from build123d import *

# Parameters (mm, degrees)
SKETCH_1_R          = 32
EXTRUDE_1_DEPTH     = 26.5
CUT_EXTRUDE_4_DEPTH = 2
SKETCH_3_R          = 26
CUT_EXTRUDE_5_DEPTH = 1
FILLET_1_R          = 10
SKETCH_4_R          = 6.68863581
CUT_EXTRUDE_6_DEPTH = 5


with BuildPart() as part:
    # 草图1 → 凸台-拉伸1 (new body)
    with BuildSketch(Plane.XY):
        Circle(SKETCH_1_R)
    extrude(amount=EXTRUDE_1_DEPTH)

    # 草图2 → 切除-拉伸4 (cut)
    with BuildSketch(Plane.XY.offset(26.5)):
        with BuildLine():
            ThreePointArc((3.045475662, 0.479690306), (3.083022023, 0), (3.045475662, -0.479690306))
            Line((3.045475662, -0.479690306), (25.683360874, -4.045364533))
            ThreePointArc((25.683360874, -4.045364533), (26, 0), (25.683360874, 4.045364533))
            Line((25.683360874, 4.045364533), (3.045475662, 0.479690306))
        make_face()
        with BuildLine():
            Line((16.34506889, -20.219760705), (1.938161822, -2.397614137))
            ThreePointArc((1.938161822, -2.397614137), (1.541511012, -2.669975393), (1.10731384, -2.877304443))
            Line((1.10731384, -2.877304443), (9.338291984, -24.265125238))
            ThreePointArc((9.338291984, -24.265125238), (13, -22.516660498), (16.34506889, -20.219760705))
        make_face()
        with BuildLine():
            Line((-9.338291984, -24.265125238), (-1.10731384, -2.877304443))
            ThreePointArc((-1.10731384, -2.877304443), (-1.541511012, -2.669975393), (-1.938161822, -2.397614137))
            Line((-1.938161822, -2.397614137), (-16.34506889, -20.219760705))
            ThreePointArc((-16.34506889, -20.219760705), (-13, -22.516660498), (-9.338291984, -24.265125238))
        make_face()
        with BuildLine():
            Line((-25.683360874, -4.045364533), (-3.045475662, -0.479690306))
            ThreePointArc((-3.045475662, -0.479690306), (-3.083022023, 0), (-3.045475662, 0.479690306))
            Line((-3.045475662, 0.479690306), (-25.683360874, 4.045364533))
            ThreePointArc((-25.683360874, 4.045364533), (-26, 0), (-25.683360874, -4.045364533))
        make_face()
        with BuildLine():
            Line((-16.34506889, 20.219760705), (-1.938161822, 2.397614137))
            ThreePointArc((-1.938161822, 2.397614137), (-1.541511012, 2.669975393), (-1.10731384, 2.877304443))
            Line((-1.10731384, 2.877304443), (-9.338291984, 24.265125238))
            ThreePointArc((-9.338291984, 24.265125238), (-13, 22.516660498), (-16.34506889, 20.219760705))
        make_face()
        with BuildLine():
            Line((9.338291984, 24.265125238), (1.10731384, 2.877304443))
            ThreePointArc((1.10731384, 2.877304443), (1.541511012, 2.669975393), (1.938161822, 2.397614137))
            Line((1.938161822, 2.397614137), (16.34506889, 20.219760705))
            ThreePointArc((16.34506889, 20.219760705), (13, 22.516660498), (9.338291984, 24.265125238))
        make_face()
    extrude(amount=-CUT_EXTRUDE_4_DEPTH, mode=Mode.SUBTRACT)

    # 草图3 → 切除-拉伸5 (cut)
    with BuildSketch(Plane.XY.offset(26.5)):
        Circle(SKETCH_3_R)
    extrude(amount=-CUT_EXTRUDE_5_DEPTH, mode=Mode.SUBTRACT)

    # 圆角1
    # the kernel refuses this fillet: 10 mm, written as the material it takes off along each edge
    with BuildSketch(Plane(origin=(0, 0, 26.5), x_dir=(1, 0, 0), z_dir=(0, -1, 0))) as fillet_1_piece_1:
        with BuildLine():
            CenterArc((22, -9.16515139), FILLET_1_R, 0, 66.421821522)
            Line((26, 0), (26.08, 0.183303028))
            ThreePointArc((26.08, 0.183303028), (29, 0.2), (32, 0.2))
            Line((32, 0.2), (32.2, 0))
            Line((32.2, 0), (32.2, -9.16515139))
            Line((32.2, -9.16515139), (32, -9.16515139))
        make_face()
    revolve(axis=Axis((0, 0, 26.5), (0, 0, 1)), mode=Mode.SUBTRACT)

    # 草图4 → 切除-拉伸6 (cut)
    with BuildSketch(Plane(origin=(0, 0, 0), x_dir=(-1, 0, 0), z_dir=(0, 0, -1))):
        Circle(SKETCH_4_R)
    extrude(amount=-CUT_EXTRUDE_6_DEPTH, mode=Mode.SUBTRACT)


solid = part.part
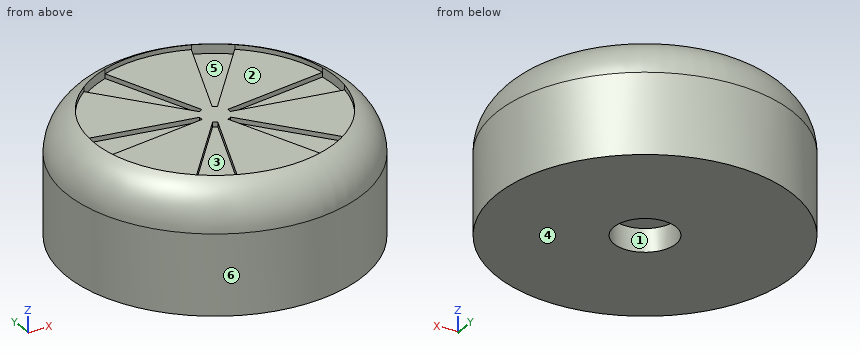
For this review, take the finished solid that the model builds, in its own axes (mm). Face numbers are marked on the shaded views. A direction names the side the tool comes from. Round coordinates to 2 decimals unless told otherwise and drop trailing zeros. Write each loop counter-clockwise with the first axis right and the second up, starting at its lowest first coordinate (ties: lowest second). Pieces come first, ordered by that corner, then holes. Notation, with made-up numbers: (-14, -39.75) - (14, -39.75) arc R31 ccw to (14, -6.75) - close; hole circle Ø3 at (-13.75, 14). An arc over 180 degrees is marked (long way). Write item = value, one per line. Start each with the question number.
1. Draft analysis for pull direction Y (two halves, no side actions). For the marked faces 3, 4, 5 and 6, state which applies: released by +Y, released by -Y, zero draft, split by the parting line, or undercut.
2. Consider section C-C on z = 4. State the section outline as (x, y) points.
3. For pin 1 Ø17 at (x, y) = (-5.5, -11) entering from +Z; pin 2 Ø12 at (y, z) = (-0.5, 11) entering from +X; pin 3 Ø1 at (y, z) = (7.5, 19.5) entering from -X; pin 4 Ø4 at (x, z) = (1, 22) entering from -Y, all flat-tipped, find the tip position at first contact; note any pin that passes through.
4. For the marked faces 1 and 2, list the 3-axis set-ups (+Z, -Z, +X, -X, +Y, -Y) from which the entire face can be reached by the end or side of a thin tool; tool diameter is ignored.
5. Consider section B-B on z = 7.5. State the section outline as (x, y) points.
6. Consider section D-D on z = 19. State the section outline as (x, y) points.
7. Consider section A-A on x = 0. State the section outline as (y, z) points, plus the area to 3 significant figures.
8. Wall thickness on L1, parallel to Y at x = 0, z = 2.1; L2, parallel to Z at x = -3, y = 12.5; L3, parallel to Z at x = -5, y = -2: over which ranges is each line inside the solid? List them lowest first.
Evaluation:
q1.face_3 = undercut
q1.face_4 = zero draft
q1.face_5 = undercut
q1.face_6 = split by the parting line
q2.outline = circle Ø64 at (0, 0); hole circle Ø13.38 at (0, 0)
q3.pin_1 = 25.5
q3.pin_2 = 32
q3.pin_3 = -31.02
q3.pin_4 = -31.63
q4.face_1 = -Z
q4.face_2 = +Z
q5.outline = circle Ø64 at (0, 0)
q6.outline = circle Ø63.72 at (0, 0)
q7.outline = (-32, 0) - (-6.69, 0) - (-6.69, 5) - (6.69, 5) - (6.69, 0) - (32, 0) - (32, 17.33) arc R10 ccw to (26, 26.5) - (26, 25.5) - (-26, 25.5) - (-26, 26.5) arc R10 ccw to (-32, 17.33) - close
q7.area = 1,550 mm2
q8.L1 = -32 to -6.69, 6.69 to 32
q8.L2 = 0 to 25.5
q8.L3 = 5 to 25.5
